```python
from build123d import *

# Parameters (mm, degrees)
SKETCH1_R                = 1.5
BOSS_EXTRUDE1_DEPTH      = 1.5
BOSS_EXTRUDE1_DEPTH_BACK = 1.5
BOSS_EXTRUDE2_DEPTH      = 5
BOSS_EXTRUDE2_DEPTH_BACK = 5


with BuildPart() as part:
    # Sketch1 → Boss-Extrude1 (new body, two sides)
    with BuildSketch(Plane(origin=(0, 0, 0), x_dir=(1, 0, 0), z_dir=(0, 1, 0))) as boss_extrude1_sk:
        with BuildLine():
            ThreePointArc((5.123475383, 2), (-5.5, 0), (5.123475383, -2))
            Line((5.123475383, -2), (24.876524617, -2))
            ThreePointArc((24.876524617, -2), (28.352990157, -5.247605032), (33.061732187, -4.569003832))
            Line((33.061732187, -4.569003832), (57.57995609, -21.641303613))
            Line((57.57995609, -21.641303613), (59.865670376, -18.358696387))
            Line((59.865670376, -18.358696387), (35.347446472, -1.286396606))
            ThreePointArc((35.347446472, -1.286396606), (31.647009843, 5.247605032), (24.876524617, 2))
            Line((24.876524617, 2), (5.123475383, 2))
        make_face()
        Circle(SKETCH1_R, mode=Mode.SUBTRACT)
        with Locations((30, 0)):
            Circle(SKETCH1_R, mode=Mode.SUBTRACT)
    extrude(amount=BOSS_EXTRUDE1_DEPTH)
    extrude(boss_extrude1_sk.sketch, amount=-BOSS_EXTRUDE1_DEPTH_BACK)

    # Sketch2 → Boss-Extrude2 (add, two sides)
    with BuildSketch(Plane(origin=(0, 0, 0), x_dir=(1, 0, 0), z_dir=(0, 1, 0))) as boss_extrude2_sk:
        Polygon((59.865670376, -18.358696387), (57.57995609, -21.641303613), (69.88973319, -30.212732185), (72.175447475, -26.930124958), align=None)
        with BuildLine():
            Line((62.399646215, -14.719550648), (59.865670376, -18.358696387))
            Line((59.865670376, -18.358696387), (72.175447475, -26.930124958))
            Line((72.175447475, -26.930124958), (74.81330558, -23.141789675))
            ThreePointArc((74.81330558, -23.141789675), (67.212824585, -20.984792896), (62.399646215, -14.719550648))
        make_face()
    extrude(amount=BOSS_EXTRUDE2_DEPTH)
    extrude(boss_extrude2_sk.sketch, amount=-BOSS_EXTRUDE2_DEPTH_BACK)


solid = part.part
```
CAD build for the part. Positions are in the model's coordinates, mm. A direction names the side the tool comes from. Give positions to 0.01 mm unless a question says otherwise; leave off trailing zeros. Order: outer loops, then holes, each group sorted by start corner. A loop starts at its lowest first (then second) coordinate and runs counter-clockwise, first axis right, second up.
(1) Mould opens along Z. For faces 3 (the flat face through (15, 0, 2)), 4 (the cylindrical face through (-5.496, 0.021, -0.213)), 5 (the cylindrical face through (28.5, -0.02, -0.07)), 6 (the cylindrical face through (67.31, 0.07, 21.05)) say: released by +Z, released by -Z, zero draft, split by the parting line, or undercut.
(2) Saw through at A-A, the plane x = 0. Give the cut face in (y, z).
(3) Saw through at D-D, the plane z = 20. Give the cut face in (x, y).
(4) Tool access for faces 1 (the flat face through (15, 0, -2)), 2 (the cylindrical face through (28.287, 0.021, 5.227)): list every direction of +Z, -Z, +X, -X, +Y, -Y with a clear straight run to the whole face (end or side of a thin tool).
(5) Flat gauge pins, fed straight in: pin 1 (8 mm diameter, centred on x = 15, z = 7, fed in from +Y); pin 2 (2.5 mm diameter, centred on x = 13.5, y = -0.5, fed in from +Z); pin 3 (0.9 mm diameter, centred on x = 10.5, y = -0.5, fed in from -Z); pin 4 (3 mm diameter, centred on y = 1, z = 12.5, fed in from -X). Where does each tip first touch, or does it go through?
(6) Saw through at C-C, the plane y = -0.5. Give the cut face in (x, z), then the cut area to 3 significant figures.
(7) Saw through at B-B, the plane z = 0. Give the cut face in (x, y), then the cut area to 3 significant figures.
(8) Drill centre lines: L1, parallel to X at y = 0.4, z = 0; L2, parallel to X at y = 1, z = 5; L3, parallel to Z at x = 0, y = 0.95. Where is each one in solid material? Low to high.
Results found:
1. face 3: released by +Z
1. face 4: split by the parting line
1. face 5: undercut
1. face 6: released by -Z
2. outline: (-1.5, -5.5) - (1.5, -5.5) - (1.5, -1.5) - (-1.5, -1.5) - close; (-1.5, 1.5) - (1.5, 1.5) - (1.5, 5.5) - (-1.5, 5.5) - close
3. outline: (55.22, -1.5) - (58.72, -1.5) - (58.72, -5) - (65.94, -5) - (65.94, 5) - (58.72, 5) - (58.72, 1.5) - (55.22, 1.5) - close
4. face 1: -Z, +Y, -Y
4. face 2: +Z, +Y, -Y
5. pin 1: passes through
5. pin 2: stops at z = 2
5. pin 3: stops at z = -2
5. pin 4: stops at x = 42.3
6. outline: (5.12, -2) - (24.88, -2) arc R5.5 ccw to (35.35, 1.29) - (59.87, 18.36) - (62.4, 14.72) arc R12.57 cw to (74.81, 23.14) - (69.89, 30.21) - (33.06, 4.57) arc R5.5 ccw to (24.88, 2) - (5.12, 2) arc R5.5 ccw (long way) to start; hole circle Ø3 at (0, 0); hole circle Ø3 at (30, 0)
6. area: 474 mm2
7. outline: (-5.5, -1.5) - (-1.5, -1.5) - (-1.5, 1.5) - (-5.5, 1.5) - close; (1.5, -1.5) - (28.5, -1.5) - (28.5, 1.5) - (1.5, 1.5) - close; (31.5, -1.5) - (35.5, -1.5) - (35.5, 1.5) - (31.5, 1.5) - close
7. area: 105 mm2
8. L1: x = -5.5 to -1.5, 1.5 to 28.5, 31.5 to 35.5
8. L2: x = -2.29 to 2.29, 27.71 to 32.29, 33.68 to 40.68
8. L3: z = -5.5 to -1.5, 1.5 to 5.5
